Could you check a few things on this model? Use its own coordinates, in mm. A direction names the side the tool comes from. Coordinates: 2 decimals unless noted, no trailing zeros. Write each loop counter-clockwise with the first axis right and the second up, starting at its lowest first coordinate (ties: lowest second). Pieces come first, ordered by that corner, then holes. Notation, with made-up numbers: (68.5, 62) - (78.5, 62) arc R30 cw to (78.5, 91) - close; hole circle Ø11 at (75, 34.5). An arc over 180 degrees is marked (long way). Answer as a JSON object with one key per item and string values. Group by question number.
1) On a 3-axis mill with a long thin cutter (end or side, diameter ignored), from which of +Z, -Z, +X, -X, +Y, -Y can I reach the whole of each face in a straight line? I mean faces 5 (the flat face through (80.4, 38.1, 36)), 6 (the cylindrical face through (64.085, 31.302, 35.014)), 7 (the flat face through (74, 43, 36)). Say none if no direction works.
2) If we section it at C-C (x = 68.5): Write out the boundary of the cut face in (y, z).
3) Please list where these lines run through material, in increasing order: line 1 along X through (y, z) = (30, 35.05); line 2 along X through (y, z) = (39, 35.2); line 3 along X through (y, z) = (38.5, 35.3).
4) We'd pull the mould along X, two halves only. Please class faces 1 (the cylindrical face through (88.643, 33.252, 35.014)), 2 (the flat face through (74, 18, 36)), 3 (the flat face through (67.6, 38.1, 36)), 4 (the flat face through (84, 27, 34)): released by +X, released by -X, zero draft, split by the parting line, or undercut.
5) If we section it at B-B (y = 34): Write out the boundary of the cut face in (x, z), plus the area to 3 significant figures.
6) Will these pins go through, and if not, where does the flat tip stop? pin 1 Ø1 at (y, z) = (29, 37.5) entering from +X; pin 2 Ø0.6 at (x, y) = (83, 39.5) entering from -Z; pin 3 Ø7.5 at (x, y) = (69.5, 39) entering from +Z.
7) If we section it at A-A (z = 34.4): Write out the boundary of the cut face in (x, y).
```python
from build123d import *

# Parameters (mm, degrees)
CYLINDER003001001005001003001001_R     = 1
CYLINDER003001001005001003001001_DEPTH = 5
CYLINDER003001001001002001001_R        = 1
CYLINDER003001001001002001001_DEPTH    = 5
CYLINDER003001001005001004001_R        = 1
CYLINDER003001001005001004001_DEPTH    = 4
CYLINDER003001001001003001_R           = 1
CYLINDER003001001001003001_DEPTH       = 4
CYLINDER003001001003001001_R           = 10
CYLINDER003001001003001001_DEPTH       = 2
CYLINDER003001001003002_R              = 15
CYLINDER003001001003002_DEPTH          = 2
CUT002005_ROLL_ANGLE                   = 180
CUT002005_PLACEMENT_ANGLE              = -90


with BuildPart() as cylinder003001001005001003001001:
    # Cylinder003001001005001003001001 → Cylinder003001001005001003001001 (new body)
    with BuildSketch(Plane(origin=(-3, -3, 26), x_dir=(1, 0, 0), z_dir=(0, 0, 1))):
        Circle(CYLINDER003001001005001003001001_R)
    extrude(amount=CYLINDER003001001005001003001001_DEPTH)


with BuildPart() as cylinder003001001001002001001:
    # Cylinder003001001001002001001 → Cylinder003001001001002001001 (new body)
    with BuildSketch(Plane(origin=(15, -3, 26), x_dir=(1, 0, 0), z_dir=(0, 0, 1))):
        Circle(CYLINDER003001001001002001001_R)
    extrude(amount=CYLINDER003001001001002001001_DEPTH)


with BuildPart() as cylinder003001001005001004001:
    # Cylinder003001001005001004001 → Cylinder003001001005001004001 (new body)
    with BuildSketch(Plane(origin=(-6.5, 6, 26), x_dir=(1, 0, 0), z_dir=(0, 0, 1))):
        Circle(CYLINDER003001001005001004001_R)
    extrude(amount=CYLINDER003001001005001004001_DEPTH)


with BuildPart() as cylinder003001001001003001:
    # Cylinder003001001001003001 → Cylinder003001001001003001 (new body)
    with BuildSketch(Plane(origin=(18.5, 6, 26), x_dir=(1, 0, 0), z_dir=(0, 0, 1))):
        Circle(CYLINDER003001001001003001_R)
    extrude(amount=CYLINDER003001001001003001_DEPTH)


with BuildPart() as fusion013001:
    # Cylinder003001001003001001 → Cylinder003001001003001001 (new body)
    with BuildSketch(Plane(origin=(6, 6, 26), x_dir=(1, 0, 0), z_dir=(0, 0, 1))):
        Circle(CYLINDER003001001003001001_R)
    extrude(amount=CYLINDER003001001003001001_DEPTH)

    # Fusion013001: union Cylinder003001001005001003001001, Cylinder003001001001002001001, Cylinder003001001005001004001, Cylinder003001001001003001
    add(cylinder003001001005001003001001.part)
    add(cylinder003001001001002001001.part)
    add(cylinder003001001005001004001.part)
    add(cylinder003001001001003001.part)


with BuildPart() as cylinder003001001003002:
    # Cylinder003001001003002 → Cylinder003001001003002 (new body)
    with BuildSketch(Plane(origin=(6, 6, 26), x_dir=(1, 0, 0), z_dir=(0, 0, 1))):
        Circle(CYLINDER003001001003002_R)
    extrude(amount=CYLINDER003001001003002_DEPTH)


with BuildPart() as sphere001001001001001001001003:
    # Sphere001001001001001001005 → Sphere001001001001001001005 (revolve)
    with BuildSketch(Plane(origin=(-3, 15, 26), x_dir=(1, 0, 0), z_dir=(0, -1, 0))):
        with BuildLine():
            ThreePointArc((0, -2.5), (1.767767, -1.767767), (2.5, 0))
            Line((2.5, 0), (0, 0))
            Line((0, 0), (0, -2.5))
        make_face()
    revolve(axis=Axis((-3, 15, 26), (0, 0, 1)))


with BuildPart() as sphere001001001001001001001006:
    # Sphere001001001001001001008 → Sphere001001001001001001008 (revolve)
    with BuildSketch(Plane(origin=(6, -6.5, 26), x_dir=(1, 0, 0), z_dir=(0, -1, 0))):
        with BuildLine():
            ThreePointArc((0, -2.5), (1.767767, -1.767767), (2.5, 0))
            Line((2.5, 0), (0, 0))
            Line((0, 0), (0, -2.5))
        make_face()
    revolve(axis=Axis((6, -6.5, 26), (0, 0, 1)))


with BuildPart() as sphere001001001001001001001004:
    # Sphere001001001001001001006 → Sphere001001001001001001006 (revolve)
    with BuildSketch(Plane(origin=(-6.5, 6, 26), x_dir=(1, 0, 0), z_dir=(0, -1, 0))):
        with BuildLine():
            ThreePointArc((0, -2.5), (1.767767, -1.767767), (2.5, 0))
            Line((2.5, 0), (0, 0))
            Line((0, 0), (0, -2.5))
        make_face()
    revolve(axis=Axis((-6.5, 6, 26), (0, 0, 1)))


with BuildPart() as sphere001001001001001001003:
    # Sphere001001001001001001003 → Sphere001001001001001001003 (revolve)
    with BuildSketch(Plane(origin=(15, -3, 26), x_dir=(1, 0, 0), z_dir=(0, -1, 0))):
        with BuildLine():
            ThreePointArc((0, -2.5), (1.767767, -1.767767), (2.5, 0))
            Line((2.5, 0), (0, 0))
            Line((0, 0), (0, -2.5))
        make_face()
    revolve(axis=Axis((15, -3, 26), (0, 0, 1)))


with BuildPart() as sphere001001001001001001001002:
    # Sphere001001001001001001004 → Sphere001001001001001001004 (revolve)
    with BuildSketch(Plane(origin=(15, 15, 26), x_dir=(1, 0, 0), z_dir=(0, -1, 0))):
        with BuildLine():
            ThreePointArc((0, -2.5), (1.767767, -1.767767), (2.5, 0))
            Line((2.5, 0), (0, 0))
            Line((0, 0), (0, -2.5))
        make_face()
    revolve(axis=Axis((15, 15, 26), (0, 0, 1)))


with BuildPart() as sphere001001001001001001001007:
    # Sphere001001001001001001001001 → Sphere001001001001001001001001 (revolve)
    with BuildSketch(Plane(origin=(6, 18.5, 26), x_dir=(1, 0, 0), z_dir=(0, -1, 0))):
        with BuildLine():
            ThreePointArc((0, -2.5), (1.767767, -1.767767), (2.5, 0))
            Line((2.5, 0), (0, 0))
            Line((0, 0), (0, -2.5))
        make_face()
    revolve(axis=Axis((6, 18.5, 26), (0, 0, 1)))


with BuildPart() as sphere001001001001001001001005:
    # Sphere001001001001001001007 → Sphere001001001001001001007 (revolve)
    with BuildSketch(Plane(origin=(18.5, 6, 26), x_dir=(1, 0, 0), z_dir=(0, -1, 0))):
        with BuildLine():
            ThreePointArc((0, -2.5), (1.767767, -1.767767), (2.5, 0))
            Line((2.5, 0), (0, 0))
            Line((0, 0), (0, -2.5))
        make_face()
    revolve(axis=Axis((18.5, 6, 26), (0, 0, 1)))


with BuildPart() as guide2:
    # Sphere001001001001001001002 → Sphere001001001001001001002 (revolve)
    with BuildSketch(Plane(origin=(-3, -3, 26), x_dir=(1, 0, 0), z_dir=(0, -1, 0))):
        with BuildLine():
            ThreePointArc((0, -2.5), (1.767767, -1.767767), (2.5, 0))
            Line((2.5, 0), (0, 0))
            Line((0, 0), (0, -2.5))
        make_face()
    revolve(axis=Axis((-3, -3, 26), (0, 0, 1)))

    # Fusion014: union Cylinder003001001003002, Sphere001001001001001001001003, Sphere001001001001001001001006, Sphere001001001001001001001004, Sphere001001001001001001003, Sphere001001001001001001001002, Sphere001001001001001001001007, Sphere001001001001001001001005
    add(cylinder003001001003002.part)
    add(sphere001001001001001001001003.part)
    add(sphere001001001001001001001006.part)
    add(sphere001001001001001001001004.part)
    add(sphere001001001001001001003.part)
    add(sphere001001001001001001001002.part)
    add(sphere001001001001001001001007.part)
    add(sphere001001001001001001001005.part)

    # Cut002005: cut Fusion013001
    add(fusion013001.part, mode=Mode.SUBTRACT)


with BuildPart() as guide2_1:
    # Cut002005 roll: moved
    add(guide2.part.rotate(Axis((0, 0, 0), (1, 0, 0)), CUT002005_ROLL_ANGLE))


with BuildPart() as guide2_2:
    # Cut002005 placement: moved
    add(guide2_1.part.moved(Location((80, 36, 62))).rotate(Axis((80, 36, 62), (0, 0, 1)), CUT002005_PLACEMENT_ANGLE))


solid = guide2_2.part
```
Here are the results:
{
 "1": {"face 5": "+Z", "face 6": "+Z, -Z", "face 7": "-Z"},
 "2": {"outline": "(16.04, 34) - (21.65, 34) - (21.65, 36) - (16.04, 36) - close; (38.35, 34) - (43.96, 34) - (43.96, 36) - (38.35, 36) - close"},
 "3": {"line 1": "x = 59 to 64, 84 to 89", "line 2": "x = 62 to 69.64, 78.36 to 82, 84 to 86", "line 3": "x = 61.64 to 68.73, 79.27 to 82.13, 83.87 to 86.36"},
 "4": {"face 1": "split by the parting line", "face 2": "undercut", "face 3": "undercut", "face 4": "zero draft"},
 "5": {"outline": "(59.54, 34) - (64.83, 34) - (64.83, 36) - (59.54, 36) - close; (83.17, 34) - (88.46, 34) - (88.46, 36) - (83.17, 36) - close", "area": "21.2 mm²"},
 "6": {"pin 1": "stops at x = 88.63", "pin 2": "stops at z = 36", "pin 3": "stops at z = 38.38"},
 "7": {"outline": "circle Ø30 at (74, 30); hole circle Ø20 at (74, 30); hole circle Ø2 at (74, 17.5); hole circle Ø2 at (74, 42.5); hole circle Ø2 at (83, 21); hole circle Ø2 at (83, 39)"}
}
